Could you check a few things on this model? Use its own coordinates, in mm. Face numbers are marked on the shaded views. A direction names the side the tool comes from. Round coordinates to 2 decimals unless told otherwise and drop trailing zeros. Write each loop counter-clockwise with the first axis right and the second up, starting at its lowest first coordinate (ties: lowest second). Pieces come first, ordered by that corner, then holes. Notation, with made-up numbers: M -33.5,54 L 18.5,54 A20 cw 18.5,65 Z; hole C 27,48 d7. An arc over 180 degrees is marked long. One line per item, written item: value. Start each with the question number.
(1) Which directions (+Z, -Z, +X, -X, +Y, -Y) give clear straight access to the entire face, cutting with the end or side of a thin tool? Please do the marked faces 4 and 5.
(2) I want a section at A-A on y = 0. Please give me the cut outline in (x, z), and give its area (3 significant figures).
(3) I'm going to push a flat-ended pin straight in: pin 1 Ø4 at (x, y) = (0, 0) entering from -Z. Where does the tip first touch, or does it pass through?
(4) Thinking about a two-plate mould opening in X: for the marked faces 1, 2 and 3, which applies, released by +X, released by -X, zero draft, split by the parting line, or undercut?
(5) If I drill on L1, parallel to X at y = 0, z = 1.1; L2, parallel to Z at x = 8.25, y = -0.25, over which ranges is the centre line in solid material (lowest first)?
```python
from build123d import *

# Parameters (mm, degrees)
F0_W     = 25
F0_H     = 25
F1_DEPTH = 7
F2_R     = 2.5
F3_DEPTH = 2
F5_DEPTH = 1
F6_R     = 1


with BuildPart() as f1:
    # F0 (on Top) → F1 (new body)
    with BuildSketch(Plane.XY):
        Rectangle(F0_W, F0_H)
    extrude(amount=F1_DEPTH)

    # F2 (on face) → F3 (cut)
    with BuildSketch(Plane(origin=(0, 0, 0), x_dir=(1, 0, 0), z_dir=(0, 0, -1))):
        Circle(F2_R)
    extrude(amount=-F3_DEPTH, mode=Mode.SUBTRACT)

    # F4 (on face) → F5 (join)
    with BuildSketch(Plane.XY.offset(7)):
        with BuildLine():
            Line((-12.5, 4.5496279283), (-0.9396926208, 0.3420201433))
            ThreePointArc((-0.9396926208, 0.3420201433), (-1, 0), (-0.9396926208, -0.3420201433))
            Line((-0.9396926208, -0.3420201433), (-12.5, -4.5496279283))
            Line((-12.5, -4.5496279283), (-4.5496279283, -12.5))
            Line((-4.5496279283, -12.5), (-0.3420201433, -0.9396926208))
            ThreePointArc((-0.3420201433, -0.9396926208), (0, -1), (0.3420201433, -0.9396926208))
            Line((0.3420201433, -0.9396926208), (4.5496279283, -12.5))
            Line((4.5496279283, -12.5), (12.5, -4.5496279283))
            Line((12.5, -4.5496279283), (0.9396926208, -0.3420201433))
            ThreePointArc((0.9396926208, -0.3420201433), (1, 0), (0.9396926208, 0.3420201433))
            Line((0.9396926208, 0.3420201433), (12.5, 4.5496279283))
            Line((12.5, 4.5496279283), (4.5496279283, 12.5))
            Line((4.5496279283, 12.5), (0.3420201433, 0.9396926208))
            ThreePointArc((0.3420201433, 0.9396926208), (0, 1), (-0.3420201433, 0.9396926208))
            Line((-0.3420201433, 0.9396926208), (-4.5496279283, 12.5))
            Line((-4.5496279283, 12.5), (-12.5, 4.5496279283))
        make_face()
    extrude(amount=F5_DEPTH)

    # F6
    f6_edges = [f1.edges().sort_by_distance(p)[0] for p in [
        (-12.5, 4.549628, 7.5),
        (-4.549628, 12.5, 7.5),
        (4.549628, 12.5, 7.5),
        (12.5, 4.549628, 7.5),
        (4.549628, -12.5, 7.5),
        (12.5, -4.549628, 7.5),
        (-4.549628, -12.5, 7.5),
        (-12.5, -4.549628, 7.5),
    ]]
    fillet(f6_edges, radius=F6_R)


solid = f1.part
```
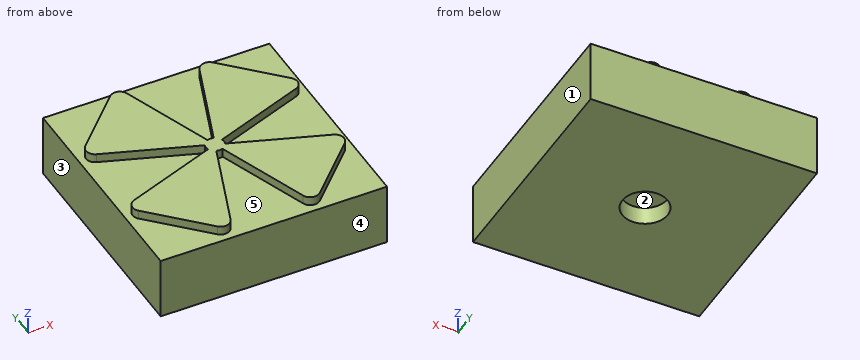
Found:
1. face 4: +Z, -Z, +X, -X, -Y
1. face 5: +Z
2. outline: M -12.5,0 L -2.5,0 L -2.5,2 L 2.5,2 L 2.5,0 L 12.5,0 L 12.5,7 L 1,7 L 1,8 L -1,8 L -1,7 L -12.5,7 Z
2. area: 167 mm²
3. pin 1: stops at z = 2
4. face 1: released by +X
4. face 2: undercut
4. face 3: released by -X
5. L1: x = -12.5 to -2.5, 2.5 to 12.5
5. L2: z = 0 to 7
